Model file for the job. Use its own axes, mm. Face numbers are marked on the shaded views. Round coordinates to 2 decimals unless told otherwise and drop trailing zeros. Loops run counter-clockwise (first coordinate to the right, second up) from the corner with the lowest first, then second, coordinate; pieces in that order, holes last. Notation, with made-up numbers: (55.5, 54) -> (63.5, 54) arc R30 ccw to (63.5, 78) -> close; hole circle Ø6 at (-2.75, -32.5). An arc over 180 degrees is marked (long way). Use a Markdown table: item, result.
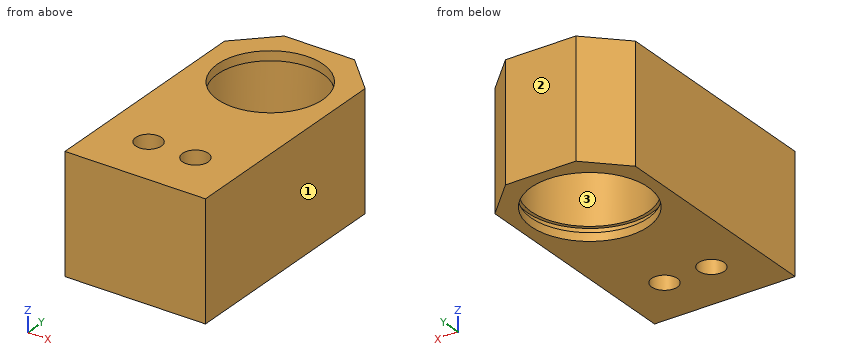
from build123d import *

# Parameters (mm, degrees)
F1_DEPTH = 50
F2_D     = 11
F3_D     = 45
F4_R     = 25
F5_DEPTH = 46
F7_START = 3.5
F6_R     = 26.5
F7_DEPTH = 2.5


with BuildPart() as f1:
    # F0 (on Top) → F1 (new body)
    with BuildSketch(Plane.XY):
        Polygon((15, 30), (-15, 30), (-30, 15), (-30, -82.5), (30, -82.5), (30, 15), align=None)
    extrude(amount=F1_DEPTH)

    # F2 (through all)
    with Locations(Plane(origin=(0, 0, 0), x_dir=(1, 0, 0), z_dir=(0, 0, -1))):
        with Locations((-10, 60), (10, 60)):
            Hole(F2_D / 2)

    # F3 (through all)
    with Locations(Plane(origin=(0, 0, 0), x_dir=(1, 0, 0), z_dir=(0, 0, -1))):
        with Locations((0, 0)):
            Hole(F3_D / 2)

    # F4 (on Top) → F5 (cut)
    with BuildSketch(Plane.XY):
        Circle(F4_R)
    extrude(amount=F5_DEPTH, mode=Mode.SUBTRACT)

    # F6 (on Top) → F7 (cut)
    with BuildSketch(Plane.XY.offset(F7_START)):
        Circle(F6_R)
    extrude(amount=F7_DEPTH, mode=Mode.SUBTRACT)


solid = f1.part
Q1. Pull direction X, two halves, no side cores. Call the marked faces 1, 2 and 3: released by +X, released by -X, zero draft, split by the parting line, or undercut.
Results list:
| item | result |
|---|---|
| face 1 | released by +X |
| face 2 | zero draft |
| face 3 | undercut |
Q2. Flat gauge pin, fed straight in: pin 1 (16 mm diameter, centred on x = 8, y = 13, fed in from -Z). Where does the tip first touch, or does it go through?
Results list:
| item | result |
|---|---|
| pin 1 | stops at z = 46 |
Q3. Drill centre lines: L1, parallel to X at y = -60, z = 11; L2, parallel to Y at x = 0, z = 49; L3, parallel to Y at x = 14, z = 17. Where is each one in solid material? Low to high. Write a range as from..to.
Results list:
| item | result |
|---|---|
| L1 | x = -30..-15.5, -4.5..4.5, 15.5..30 |
| L2 | y = -82.5..-22.5, 22.5..30 |
| L3 | y = -82.5..-63.77, -56.23..-20.71, 20.71..30 |
Q4. Band-saw the part on B-B, the plane y = -60. Give the cut face in (x, z).
Results list:
| item | result |
|---|---|
| outline | (-30, 0) -> (-15.5, 0) -> (-15.5, 50) -> (-30, 50) -> close; (-4.5, 0) -> (4.5, 0) -> (4.5, 50) -> (-4.5, 50) -> close; (15.5, 0) -> (30, 0) -> (30, 50) -> (15.5, 50) -> close |
Q5. Band-saw the part on A-A, the plane x = 0. Give the cut face in (y, z).
Results list:
| item | result |
|---|---|
| outline | (-82.5, 0) -> (-25, 0) -> (-25, 3.5) -> (-26.5, 3.5) -> (-26.5, 6) -> (-25, 6) -> (-25, 46) -> (-22.5, 46) -> (-22.5, 50) -> (-82.5, 50) -> close; (22.5, 46) -> (25, 46) -> (25, 6) -> (26.5, 6) -> (26.5, 3.5) -> (25, 3.5) -> (25, 0) -> (30, 0) -> (30, 50) -> (22.5, 50) -> close |
Q6. Band-saw the part on C-C, the plane y = 0. Give the cut face in (x, z).
Results list:
| item | result |
|---|---|
| outline | (-30, 0) -> (-25, 0) -> (-25, 3.5) -> (-26.5, 3.5) -> (-26.5, 6) -> (-25, 6) -> (-25, 46) -> (-22.5, 46) -> (-22.5, 50) -> (-30, 50) -> close; (22.5, 46) -> (25, 46) -> (25, 6) -> (26.5, 6) -> (26.5, 3.5) -> (25, 3.5) -> (25, 0) -> (30, 0) -> (30, 50) -> (22.5, 50) -> close |
Q7. Band-saw the part on D-D, the plane z = 12.5. Give the cut face in (x, y).
Results list:
| item | result |
|---|---|
| outline | (-30, -82.5) -> (30, -82.5) -> (30, 15) -> (15, 30) -> (-15, 30) -> (-30, 15) -> close; hole circle Ø50 at (0, 0); hole circle Ø11 at (-10, -60); hole circle Ø11 at (10, -60) |
